from build123d import *

# Parameters (mm, degrees)
SKETCH2_R           = 4.1
BOSS_EXTRUDE1_DEPTH = 3
FILLET1_RADIUS      = 6.25
FILLET1_LENGTH      = 6
FILLET2_R           = 2
SKETCH3_R           = 1.1
CUT_EXTRUDE1_DEPTH  = 3


with BuildPart() as part:
    # Sketch2 → Boss-Extrude1 (new, symmetric)
    with BuildSketch(Plane.XY):
        Polygon((6.25, -6.5), (15, -6.5), (15, -9.5), (-15, -9.5), (-15, -6.5), (-6.25, -6.5), (-6.25, 6.1), (6.25, 6.1), align=None)
        Circle(SKETCH2_R, mode=Mode.SUBTRACT)
    extrude(amount=BOSS_EXTRUDE1_DEPTH, both=True)

    # Fillet1: full round fillet: the end face becomes a half cylinder, R = half its width
    fillet1_face = Plane((0, 6.1, 0), x_dir=(0, 0, 1), z_dir=(0, 1, 0))  # on the end face: x along it, z out of the body
    fillet1_slab = fillet1_face.offset(-FILLET1_RADIUS / 2) * Box(FILLET1_LENGTH, 2 * FILLET1_RADIUS, FILLET1_RADIUS, mode=Mode.PRIVATE)  # the body's end, R deep
    fillet1_round = Plane((0, -0.15, 0), x_dir=(0, 1, 0), z_dir=(0, 0, 1)) * Cylinder(FILLET1_RADIUS, FILLET1_LENGTH, mode=Mode.PRIVATE)  # its axis R under the face
    add(fillet1_slab - fillet1_round, mode=Mode.SUBTRACT)

    # Fillet2
    fillet2_edges = [part.edges().sort_by_distance(p)[0] for p in [
        (6.25, -6.5, 0),
        (-6.25, -6.5, 0),
    ]]
    fillet(fillet2_edges, radius=FILLET2_R)

    # Sketch3 → Cut-Extrude1 (cut)
    with BuildSketch(Plane(origin=(0, -6.5, 0), x_dir=(1, 0, 0), z_dir=(0, 1, 0))):
        with Locations(Location((-11, 0, 0), (0, 0, 180))):
            Circle(SKETCH3_R)
        with Locations(Location((11, 0, 0), (0, 0, 180))):
            Circle(SKETCH3_R)
    extrude(amount=-CUT_EXTRUDE1_DEPTH, mode=Mode.SUBTRACT)


solid = part.part
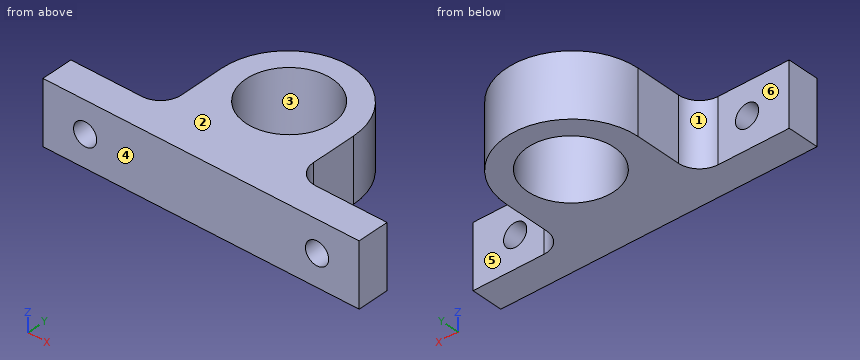
Could you check a few things on this model? Use its own coordinates, in mm. Face numbers are marked on the shaded views. A direction names the side the tool comes from. Give positions to 0.01 mm unless a question says otherwise; leave off trailing zeros. Loops run counter-clockwise (first coordinate to the right, second up) from the corner with the lowest first, then second, coordinate; pieces in that order, holes last. Notation, with made-up numbers: M 78,21 L 99,21 A21 cw 99,53 Z; hole C -36.5,-3 d11. An arc over 180 degrees is marked long. Answer as a JSON object with one key per item and string values.
Q1. For P1, Ø3.5, axis at x = 11, z = 0, coming from the +Y side; P2, Ø2, axis at y = 3, z = 0, coming from the +X side; P3, Ø1.5, axis at y = 3, z = 1.5, coming from the +X side; P4, Ø1.8, axis at x = -11, z = 0, coming from the +Y side, each with a flat end and sliding along its axis, tell me the tip position at first contact or that it passes through.
Values found:
{"P1": "stops at y = -6.5", "P2": "stops at x = 5.87", "P3": "stops at x = 5.77", "P4": "passes through"}
Q2. If we mould it in two halves opening along Y, with no side actions, what happens to the marked faces 1, 2 and 3? For each: pulls with the +Y half, pulls with the -Y half, needs draft (parallel to the pull), parting line crosses it, or undercut.
Values found:
{"face 1": "pulls with the +Y half", "face 2": "needs draft", "face 3": "undercut"}
Q3. Suppose I cut it at C-C, the plane z = 1.8. List the corners of the cut face in (x, y) for me, plus the area to 3 significant figures.
Values found:
{"outline": "M -15,-9.5 L 15,-9.5 L 15,-6.5 L 8.25,-6.5 A2 cw 6.25,-4.5 L 6.25,-0.15 A6.25 ccw -6.25,-0.15 L -6.25,-4.5 A2 cw -8.25,-6.5 L -15,-6.5 Z; hole C 0,0 d8.2", "area": "180 mm²"}
Q4. For the marked faces 4, 5 and 6, which set-ups out of +Z, -Z, +X, -X, +Y, -Y let a thin tool reach every point of the face, with its end or its side?
Values found:
{"face 4": "+Z, -Z, +X, -X, -Y", "face 5": "+Z, -Z, +X, +Y", "face 6": "+Z, -Z, -X, +Y"}
Q5. Suppose I cut it at D-D, the plane y = -1.75. List the corners of the cut face in (x, z) for me, plus the area to 3 significant figures.
Values found:
{"outline": "M -6.25,-3 L -3.71,-3 L -3.71,3 L -6.25,3 Z; M 3.71,-3 L 6.25,-3 L 6.25,3 L 3.71,3 Z", "area": "30.5 mm²"}
Q6. Suppose I cut it at A-A, the plane x = 0. List the corners of the cut face in (y, z) for me.
Values found:
{"outline": "M -9.5,-3 L -4.1,-3 L -4.1,3 L -9.5,3 Z; M 4.1,-3 L 6.1,-3 L 6.1,3 L 4.1,3 Z"}
Q7. If I drill on probe 1 along Z at (x, y) = (11, -7.25); probe 2 along Y at (x, z) = (0, -0.8); probe 3 along X at (y, z) = (-7.5, 0.6), over which ranges is the centre line in solid material (lowest first)? Write a range as [from, to].
Values found:
{"probe 1": "z = [-3, -1.1], [1.1, 3]", "probe 2": "y = [-9.5, -4.1], [4.1, 6.1]", "probe 3": "x = [-15, -11.92], [-10.08, 10.08], [11.92, 15]"}
Q8. Suppose I cut it at B-B, the plane z = 0. List the corners of the cut face in (x, y) for me, plus the area to 3 significant figures.
Values found:
{"outline": "M -15,-9.5 L -12.1,-9.5 L -12.1,-6.5 L -15,-6.5 Z; M -9.9,-9.5 L 9.9,-9.5 L 9.9,-6.5 L 8.25,-6.5 A2 cw 6.25,-4.5 L 6.25,-0.15 A6.25 ccw -6.25,-0.15 L -6.25,-4.5 A2 cw -8.25,-6.5 L -9.9,-6.5 Z; M 12.1,-9.5 L 15,-9.5 L 15,-6.5 L 12.1,-6.5 Z; hole C 0,0 d8.2", "area": "166 mm²"}
